Input: part model. Units: mm. Frame: model coordinates. A direction names the side the tool comes from. Round coordinates to 2 decimals unless told otherwise and drop trailing zeros. Loops run counter-clockwise (first coordinate to the right, second up) from the corner with the lowest first, then second, coordinate; pieces in that order, holes last. Notation, with made-up numbers: M 76.25,-3.5 L 97.25,-3.5 A13 cw 97.25,3.5 Z; hole C 50.25,18 d11. An arc over 180 degrees is marked long. Put each result on its own line as item: value. Start each with the question number.
1) Section B-B on x = -10.75. Output: boundary loops of the cut face in (y, z).
2) Reachability of faces 4 (the face through (-8.26, 6.33, 7.6)), 5 (the face through (-12, 3.5, 3)), 6 (the face through (-3, 0, 8.5)), 7 (the face through (-2, -6.5, 11)) from +Z, -Z, +X, -X, +Y, -Y: full face, straight path, thin tool, end or side. Return the list, or none.
3) Section C-C on z = 6. Output: boundary loops of the cut face in (x, y), plus the area to 3 significant figures.
4) Draft query along Y for faces 1 (the face through (-4, 13.5, 3)), 2 (the face through (3.14, -8.86, 20.99)), 3 (the face through (3.49, -0.08, 22.42)). Return one class per face: +Y half, -Y half, draft (parallel to the pull), parting line (faces both ways), or undercut.
5) Line query: probe 1 along Z at (x, y) = (-10, 3.5); probe 2 along Z at (x, y) = (-4.5, 3.5); probe 3 along X at (y, z) = (8, 22). Output: solid intervals per line, ascending.
6) Section A-A on y = 8.75. Output: boundary loops of the cut face in (x, z).
7) Section D-D on y = -9.25. Output: boundary loops of the cut face in (x, z), plus the area to 3 significant figures.
8) Pin query (flat end, axial travel): pin 1 (3 mm diameter, centred on x = 2, y = -1.5, fed in from -Z); pin 2 (1.2 mm diameter, centred on x = -4.5, y = 8, fed in from -Z); pin 3 (0.8 mm diameter, centred on x = -12, z = 3.5, fed in from -Y). Return the tip coordinate at first contact, or that it passes through.
from build123d import *

# Parameters (mm, degrees)
BOSS_EXTRUDE1_DEPTH      = 5
BOSS_EXTRUDE1_DEPTH_BACK = 5
SKETCH2_W                = 3.7
SKETCH2_H                = 10
BOSS_EXTRUDE2_DEPTH      = 1
SKETCH3_W                = 1
SKETCH3_H                = 10
BOSS_EXTRUDE3_DEPTH      = 1.5
SKETCH4_W                = 6.7
SKETCH4_H                = 27
SKETCH4_W_2              = 1.5
BOSS_EXTRUDE4_DEPTH      = 1.5
SKETCH5_W                = 4
SKETCH5_H                = 13
BOSS_EXTRUDE5_DEPTH      = 2.7
CUT_EXTRUDE1_DEPTH       = 29.339724769
BOSS_EXTRUDE6_START      = -1.5
BOSS_EXTRUDE6_DEPTH      = 8
CUT_EXTRUDE2_START       = -3.25
SKETCH8_W                = 4.8
SKETCH8_H                = 6.5
CUT_EXTRUDE2_DEPTH       = 3.25
FILLET4_R                = 1
CHAMFER1_SIZE            = 2
CHAMFER3_SIZE            = 0.5
SKETCH4_3_W              = 1
SKETCH4_3_H              = 27
BOSS_EXTRUDE7_DEPTH      = 2
SKETCH4_4_W              = 1
SKETCH4_4_H              = 27
BOSS_EXTRUDE8_DEPTH      = 1.5
FILLET6_R                = 1
FILLET8_R                = 0.4
SKETCH9_R                = 9.5
CUT_EXTRUDE3_DEPTH       = 32.948239388


with BuildPart() as part:
    # Sketch1 → Boss-Extrude1 (new, two sides: drawn at the far end of the back side and taken through both)
    with BuildSketch(Plane(origin=(0, 0, 0), x_dir=(1, 0, 0), z_dir=(0, 1, 0)).offset(-BOSS_EXTRUDE1_DEPTH_BACK)):
        Polygon((0, 0), (-2.2, 0), (-2.2, -1.270170592), align=None)
    extrude(amount=BOSS_EXTRUDE1_DEPTH + BOSS_EXTRUDE1_DEPTH_BACK)

    # Sketch2 → Boss-Extrude2 (add)
    with BuildSketch(Plane(origin=(0, 0, 0), x_dir=(-1, 0, 0), z_dir=(0, 0, -1))):
        with Locations((1.85, 0)):
            Rectangle(SKETCH2_W, SKETCH2_H)
    extrude(amount=BOSS_EXTRUDE2_DEPTH)

    # Sketch3 → Boss-Extrude3 (add)
    with BuildSketch(Plane.ZY.offset(3.7)):
        Polygon((0, -5), (0, -13.5), (22.5, -13.5), (22.5, 13.5), (0, 13.5), (0, 5), align=None)
        with Locations((-0.5, 0)):
            Rectangle(SKETCH3_W, SKETCH3_H)
    extrude(amount=BOSS_EXTRUDE3_DEPTH)

    # Sketch4 → Boss-Extrude4 (add)
    with BuildSketch(Plane.XY.offset(22.5)):
        with Locations((-0.35, 0)):
            Rectangle(SKETCH4_W, SKETCH4_H)
        with Locations((-4.45, 0)):
            Rectangle(SKETCH4_W_2, SKETCH4_H)
    extrude(amount=BOSS_EXTRUDE4_DEPTH)

    # Sketch5 → Boss-Extrude5 (add)
    with BuildSketch(Plane(origin=(-3.7, 0, 0), x_dir=(0, 0, -1), z_dir=(1, 0, 0))):
        with Locations((-10.5, 0)):
            Rectangle(SKETCH5_W, SKETCH5_H)
    extrude(amount=BOSS_EXTRUDE5_DEPTH)

    # Sketch7 → Cut-Extrude1 (cut, through all)
    with BuildSketch(Plane(origin=(-3.7, 0, 0), x_dir=(0, 0, -1), z_dir=(1, 0, 0))):
        with BuildLine():
            Line((-5.25, 5.08113883), (-5.25, 13.5))
            Line((-5.25, 13.5), (-6.75, 13.5))
            Line((-6.75, 13.5), (-6.75, 5.08113883))
            ThreePointArc((-6.75, 5.08113883), (-6, 1.75), (-5.25, 5.08113883))
        make_face()
    extrude(amount=-CUT_EXTRUDE1_DEPTH, mode=Mode.SUBTRACT)

    # Sketch7<3> → Boss-Extrude6 (add)
    with BuildSketch(Plane(origin=(-3.7, 0, 0), x_dir=(0, 0, -1), z_dir=(1, 0, 0)).offset(BOSS_EXTRUDE6_START)):
        with BuildLine():
            Line((-8.5, 1.423344034), (-8.5, 5.576655966))
            ThreePointArc((-8.5, 5.576655966), (-9.25, 3.5), (-8.5, 1.423344034))
        make_face()
        with BuildLine():
            Line((-6.75, 5.08113883), (-6.75, 6.66227766))
            ThreePointArc((-6.75, 6.66227766), (-7.713262565, 6.261744265), (-8.5, 5.576655966))
            Line((-8.5, 5.576655966), (-8.5, 1.423344034))
            ThreePointArc((-8.5, 1.423344034), (-4.896029892, 0.443245185), (-2.75, 3.5))
            ThreePointArc((-2.75, 3.5), (-3.450490243, 5.515564437), (-5.25, 6.66227766))
            Line((-5.25, 6.66227766), (-5.25, 5.08113883))
            ThreePointArc((-5.25, 5.08113883), (-4.520980054, 4.435414347), (-4.25, 3.5))
            ThreePointArc((-4.25, 3.5), (-6.935414347, 2.020980054), (-6.75, 5.08113883))
        make_face()
    extrude(amount=-BOSS_EXTRUDE6_DEPTH)

    # Sketch8 → Cut-Extrude2 (cut)
    with BuildSketch(Plane(origin=(0, 0.25, 0), x_dir=(-1, 0, 0), z_dir=(0, -1, 0)).offset(CUT_EXTRUDE2_START)):
        with Locations((10.8, -6)):
            Rectangle(SKETCH8_W, SKETCH8_H)
    extrude(amount=CUT_EXTRUDE2_DEPTH, mode=Mode.SUBTRACT)

    # Fillet4
    fillet4_edges = [part.edges().sort_by_distance(p)[0] for p in [
        (-1, 0, 8.5),
        (-1, 0, 12.5),
    ]]
    fillet(fillet4_edges, radius=FILLET4_R)

    # Chamfer1
    # the kernel refuses this chamfer: 2 mm, written as the material it adds along each edge
    with BuildSketch(Plane(origin=(-8.4, 3.5, -2.393365976), x_dir=(0.027495876610586487, -0.9996219169112968, 0), z_dir=(0, 0, 1))) as chamfer1_piece_1_section:
        Polygon((CHAMFER1_SIZE * 0.999621916911, -CHAMFER1_SIZE * 0.0274958766106), (-CHAMFER1_SIZE * 0.0274958766106, -CHAMFER1_SIZE * 0.999621916911), (0, 0), align=None)
    chamfer1_piece_1 = extrude(amount=11.786731952, mode=Mode.PRIVATE)
    chamfer1_piece_1 = chamfer1_piece_1 - Plane(origin=(-8.681951998, 3.5, 6), x_dir=(0, 0.9035079029052511, -0.4285714285714289), z_dir=(1, 0, 0)) * Cylinder(1.75, 32, mode=Mode.PRIVATE)
    chamfer1_piece_1 = chamfer1_piece_1 & Plane(origin=(-8.681951998, 3.5, 6), x_dir=(0, 0.6389710663783268, 0.7692307692307582), z_dir=(1, 0, 0)) * Cylinder(3.25, 32, mode=Mode.PRIVATE)
    add(chamfer1_piece_1)
    with BuildSketch(Plane(origin=(-8.4, 3.5, 2.606634024), x_dir=(-0.9996219169112968, 0.02749587661058627, 0), z_dir=(0, 0, 1))) as chamfer1_piece_2_section:
        Polygon((CHAMFER1_SIZE * 0.999621916911, CHAMFER1_SIZE * 0.0274958766106), (-CHAMFER1_SIZE * 0.0274958766106, CHAMFER1_SIZE * 0.999621916911), (0, 0), align=None)
    chamfer1_piece_2 = extrude(amount=11.786731952, mode=Mode.PRIVATE)
    chamfer1_piece_2 = chamfer1_piece_2 - Plane(origin=(-10.090710098, 3.5, 6), x_dir=(0, 0.9035079029052511, -0.4285714285714289), z_dir=(1, 0, 0)) * Cylinder(1.75, 32, mode=Mode.PRIVATE)
    chamfer1_piece_2 = chamfer1_piece_2 & Plane(origin=(-10.090710098, 3.5, 6), x_dir=(0, 0.6389710663783268, 0.7692307692307582), z_dir=(1, 0, 0)) * Cylinder(3.25, 32, mode=Mode.PRIVATE)
    add(chamfer1_piece_2)

    # Chamfer3
    chamfer3_edges = [part.edges().sort_by_distance(p)[0] for p in [
        (-3.7, 1.75, 6),
    ]]
    chamfer(chamfer3_edges, length=CHAMFER3_SIZE)



with BuildPart() as body_2:
    # Sketch4<3> → Boss-Extrude7 (new body)
    with BuildSketch(Plane.XY.offset(22.5)):
        with Locations((3.5, 0)):
            Rectangle(SKETCH4_3_W, SKETCH4_3_H)
    extrude(amount=-BOSS_EXTRUDE7_DEPTH)


with BuildPart() as part_1:
    add(part.part)

    add(body_2.part)  # Boss-Extrude8 merges body 2
    # Sketch4<4> → Boss-Extrude8 (add)
    with BuildSketch(Plane.XY.offset(22.5)):
        with Locations((3.5, 0)):
            Rectangle(SKETCH4_4_W, SKETCH4_4_H)
        with Locations((3.5, 0)):
            Rectangle(SKETCH4_4_W, SKETCH4_4_H)
        with Locations((3.5, 0)):
            Rectangle(SKETCH4_4_W, SKETCH4_4_H)
    extrude(amount=BOSS_EXTRUDE8_DEPTH)

    # Fillet6
    # the kernel refuses this fillet: 1 mm, written as the material it takes off along each edge
    with BuildSketch(Plane(origin=(6.5, -13.5, 20.5), x_dir=(0, 0, 1), z_dir=(-1, 0, 0))) as fillet6_piece_1:
        with BuildLine():
            CenterArc((FILLET6_R, FILLET6_R), FILLET6_R, 180, 90)
            Line((0, FILLET6_R), (0, 0))
            Line((0, 0), (FILLET6_R, 0))
        make_face()
    extrude(amount=6, mode=Mode.SUBTRACT)
    with BuildSketch(Plane(origin=(4, 16, 20.5), x_dir=(-1, 0, 0), z_dir=(0, -1, 0))) as fillet6_piece_2:
        with BuildLine():
            CenterArc((FILLET6_R, -FILLET6_R), FILLET6_R, 90, 90)
            Line((0, -FILLET6_R), (0, 0))
            Line((0, 0), (FILLET6_R, 0))
        make_face()
    extrude(amount=32, mode=Mode.SUBTRACT)
    with BuildSketch(Plane(origin=(3, -16, 20.5), x_dir=(0, 0, 1), z_dir=(0, 1, 0))) as fillet6_piece_3:
        with BuildLine():
            CenterArc((FILLET6_R, FILLET6_R), FILLET6_R, 180, 90)
            Line((0, FILLET6_R), (0, 0))
            Line((0, 0), (FILLET6_R, 0))
        make_face()
    extrude(amount=32, mode=Mode.SUBTRACT)
    with BuildSketch(Plane(origin=(0.5, 13.5, 20.5), x_dir=(0, -1, 0), z_dir=(1, 0, 0))) as fillet6_piece_4:
        with BuildLine():
            CenterArc((FILLET6_R, -FILLET6_R), FILLET6_R, 90, 90)
            Line((0, -FILLET6_R), (0, 0))
            Line((0, 0), (FILLET6_R, 0))
        make_face()
    extrude(amount=6, mode=Mode.SUBTRACT)

    # Fillet8
    fillet8_edges = [part_1.edges().sort_by_distance(p)[0] for p in [
        (4, 0, 24),
        (0, 0, -1),
        (-5.2, 9.25, 0),
        (-5.2, -9.25, 0),
        (-5.2, 0, -1),
        (-5.2, 0, 24),
    ]]
    fillet(fillet8_edges, radius=FILLET8_R)

    # Sketch9 → Cut-Extrude3 (cut, through all)
    with BuildSketch(Plane.ZY.offset(-3)):
        with Locations((12.921330644, 0)):
            Circle(SKETCH9_R)
    extrude(amount=-CUT_EXTRUDE3_DEPTH, mode=Mode.SUBTRACT)


solid = part_1.part
Geometry results:
1. outline: M 3.5,2.75 A3.25 ccw 6.66,5.25 L 5.08,5.25 A1.75 cw 3.5,4.25 Z; M 3.5,7.75 A1.75 cw 5.08,6.75 L 6.66,6.75 A3.25 ccw 3.5,9.25 Z
2. face 4: -X
2. face 5: +Z, -Z, -X, -Y
2. face 6: +X, +Y, -Y
2. face 7: -Z, +X, -Y
3. outline: M -8.65,1.75 L -8.4,1.5 L -8.4,0.25 L -5.2,0.25 L -5.2,-13.5 L -3.7,-13.5 L -3.7,1.25 L -4.2,1.75 Z
3. area: 27.6 mm²
4. face 1: +Y half
4. face 2: draft
4. face 3: undercut
5. probe 1: z = 2.75 to 4.25, 7.75 to 9.25
5. probe 2: z = -1 to 4.25, 7.75 to 24
5. probe 3: x = -5.2 to -3.7, 3 to 4
6. outline: M -5.2,0.4 A0.4 ccw -4.8,0 L -3.7,0 L -3.7,5.25 L -5.2,5.25 Z; M -5.2,6.75 L -3.7,6.75 L -3.7,22.5 L 3,22.5 L 3,21.5 A1 ccw 3.5,20.63 A1 ccw 4,21.5 L 4,23.6 A0.4 ccw 3.6,24 L -4.8,24 A0.4 ccw -5.2,23.6 Z
7. outline: M -5.2,0.4 A0.4 ccw -4.8,0 L -3.7,0 L -3.7,22.5 L 3,22.5 L 3,21.5 A1 ccw 3.5,20.63 A1 ccw 4,21.5 L 4,23.6 A0.4 ccw 3.6,24 L -4.8,24 A0.4 ccw -5.2,23.6 Z
7. area: 49.1 mm²
8. pin 1: stops at z = 22.05
8. pin 2: stops at z = 0
8. pin 3: stops at y = 3.5
